Source: three-view drawing plus pictorial views. Frame: mm from the lowest corner of the part. Coordinates: 2 decimals unless noted, no trailing zeros. Order: outer loops, then holes, each group sorted by start corner. A loop starts at its lowest first (then second) coordinate and runs counter-clockwise, first axis right, second up. Notation, with made-up numbers: (12.5, 85) -> (62.5, 85) arc R14 ccw to (62.5, 89) -> close; hole circle Ø9 at (30, -27.75). An arc over 180 degrees is marked (long way). Use CSV: the item, a comma, the result in double quotes. Start each with the question number.
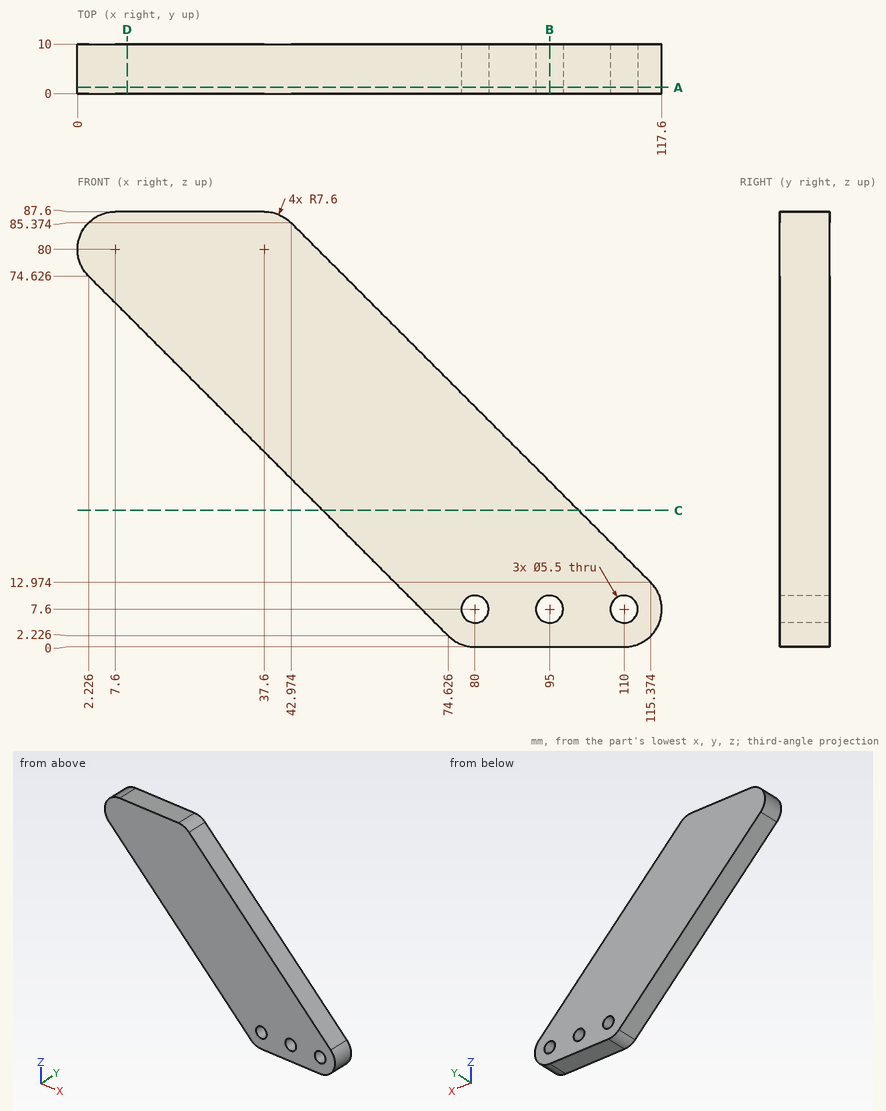
1. Section B-B on x = 95. Return loops of the section in (y, z).
2. Contact query for flat-ended pins moving along their axis: P1, Ø3, axis at y = 5, z = 28, coming from the +X side; P2, Ø5, axis at x = 26, y = 2, coming from the -Z side; P3, Ø1, axis at x = 77.5, y = 2, coming from the +Z side. Output: stop coordinate, or through.
3. Section C-C on z = 27.5. Return loops of the section in (x, y).
4. Material intervals for line 1 along Z through (x, y) = (95, 4.5); line 2 along X through (y, z) = (6, 64.5); line 3 along Z through (x, y) = (80, 6.75), sorted ascending.
5. Section D-D on x = 10. Return loops of the section in (y, z), then the cut area to 3 significant figures.
6. Section A-A on y = 1.25. Return loops of the section in (x, z).
Values follow:
1,outline,"(0, 0) -> (10, 0) -> (10, 4.85) -> (0, 4.85) -> close; (0, 10.35) -> (10, 10.35) -> (10, 33.35) -> (0, 33.35) -> close"
2,P1,"stops at x = 101.85"
2,P2,"stops at z = 48.35"
2,P3,"stops at z = 51.35"
3,outline,"(49.35, 0) -> (100.85, 0) -> (100.85, 10) -> (49.35, 10) -> close"
4,line 1,"z = 0 to 4.85, 10.35 to 33.35"
4,line 2,"x = 12.35 to 63.85"
4,line 3,"z = 0 to 4.85, 10.35 to 48.35"
5,outline,"(0, 66.85) -> (10, 66.85) -> (10, 87.6) -> (0, 87.6) -> close"
5,area,"207 mm2"
6,outline,"(2.23, 74.63) -> (74.63, 2.23) arc R7.6 ccw to (80, 0) -> (110, 0) arc R7.6 ccw to (115.37, 12.97) -> (42.97, 85.37) arc R7.6 ccw to (37.6, 87.6) -> (7.6, 87.6) arc R7.6 ccw to start; hole circle Ø5.5 at (80, 7.6); hole circle Ø5.5 at (95, 7.6); hole circle Ø5.5 at (110, 7.6)"
